Design review of the part built by this model. Coordinates are the model's own, in mm. Give positions to 0.01 mm unless a question says otherwise; leave off trailing zeros. Write each loop counter-clockwise with the first axis right and the second up, starting at its lowest first coordinate (ties: lowest second). Pieces come first, ordered by that corner, then holes.
```python
from build123d import *

# Parameters (mm, degrees)
SKETCH1_R           = 3.175
BOSS_EXTRUDE2_DEPTH = 5.4102
CUT_EXTRUDE1_DEPTH  = 5.4102


with BuildPart() as part:
    # Sketch1 → Boss-Extrude2 (new body)
    with BuildSketch(Plane(origin=(0, 0, 0), x_dir=(0, 0, -1), z_dir=(1, 0, 0))):
        with BuildLine():
            ThreePointArc((109.510185389, -69.196321406), (62.517678, -113.455504659), (0, -129.54))
            Line((0, -129.54), (50.929375256, -129.54))
            ThreePointArc((50.929375256, -129.54), (115.029071249, -78.375542305), (139.192, 0))
            Line((139.192, 0), (129.54, 0))
            ThreePointArc((129.54, 0), (124.431830765, -36.01848265), (109.510185389, -69.196321406))
        make_face()
        with BuildLine():
            ThreePointArc((116.979702463, -71.909902638), (112.921896515, -74.959702412), (111.120629291, -70.213914368))
            ThreePointArc((111.120629291, -70.213914368), (114.68750841, -68.860102864), (116.979702463, -71.909902638))
        make_face(mode=Mode.SUBTRACT)
        with Locations((133.35, -12.7)):
            Circle(SKETCH1_R, mode=Mode.SUBTRACT)
    extrude(amount=BOSS_EXTRUDE2_DEPTH)

    # Sketch2 → Cut-Extrude1 (cut)
    with BuildSketch(Plane(origin=(5.4102, 0, 0), x_dir=(0, 0, -1), z_dir=(1, 0, 0))):
        Polygon((139.192, 0), (129.268805309, -8.37780246), (129.54, 0), align=None)
    extrude(amount=-CUT_EXTRUDE1_DEPTH, mode=Mode.SUBTRACT)


solid = part.part
```
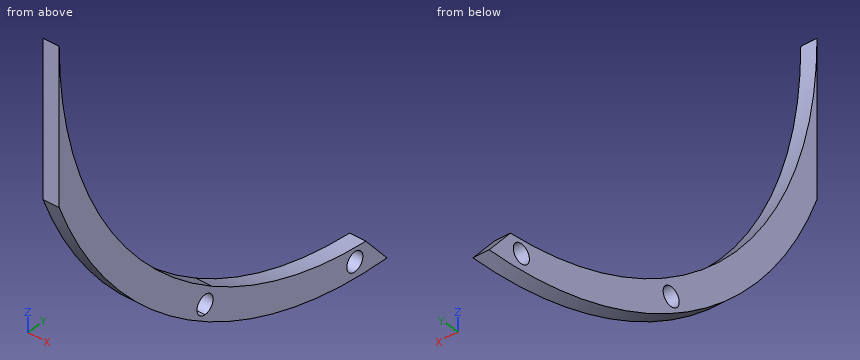
(1) Consider section C-C, the plane z = -133.35. Give the boundary of the cut face in (x, y) (3 decimals).
Resolved:
outline: (0, -39.902) - (5.41, -39.902) - (5.41, -15.875) - (0, -15.875) - close; (0, -9.525) - (5.41, -9.525) - (5.41, -4.932) - (0, -4.932) - close
(2) Clearance check with flat-ended pins moving along their axes: P1, Ø2, axis at x = 1, y = -90.5, coming from the -Z side; P2, Ø1, axis at x = 3.5, z = -94.5, coming from the +Y side; P3, Ø1, axis at x = 4.5, y = -51.5, coming from the -Z side. State where each tip first meets the part, or that it passes through.
Resolved:
P1: stops at z = -106.6
P2: stops at y = -88.07
P3: stops at z = -129.51
(3) Consider section D-D, the plane z = -47. Give the boundary of the cut face in (x, y).
Resolved:
outline: (0, -129.54) - (5.41, -129.54) - (5.41, -120.71) - (0, -120.71) - close
(4) Consider section B-B, the plane y = -12.7. Give the boundary of the cut face in (x, z) (3 decimals).
Resolved:
outline: (0, -138.611) - (5.41, -138.611) - (5.41, -136.525) - (0, -136.525) - close; (0, -130.175) - (5.41, -130.175) - (5.41, -128.916) - (0, -128.916) - close
(5) To check wall thickness, follow L1, parallel to Z at x = 3.85, y = -12; L2, parallel to Y at x = 4.3, z = -47; L3, parallel to Z at x = 1.25, y = -52. State the ranges of each line that lie inside material, in increasing order.
Resolved:
L1: z = -138.67 to -136.45, -130.25 to -128.98
L2: y = -129.54 to -120.71
L3: z = -129.11 to -118.64
(6) Consider section A-A, the plane x = 4.1. Give the boundary of the cut face in (y, z) (3 decimals), then the cut area to 3 significant figures.
Resolved:
outline: (-129.54, -50.929) arc R139.192 ccw to (0, -139.192) - (-8.378, -129.269) arc R129.54 cw to (-129.54, 0) - close; hole circle Ø6.35 at (-71.91, -113.805); hole circle Ø6.35 at (-12.7, -133.35)
area: 1,600 mm2
